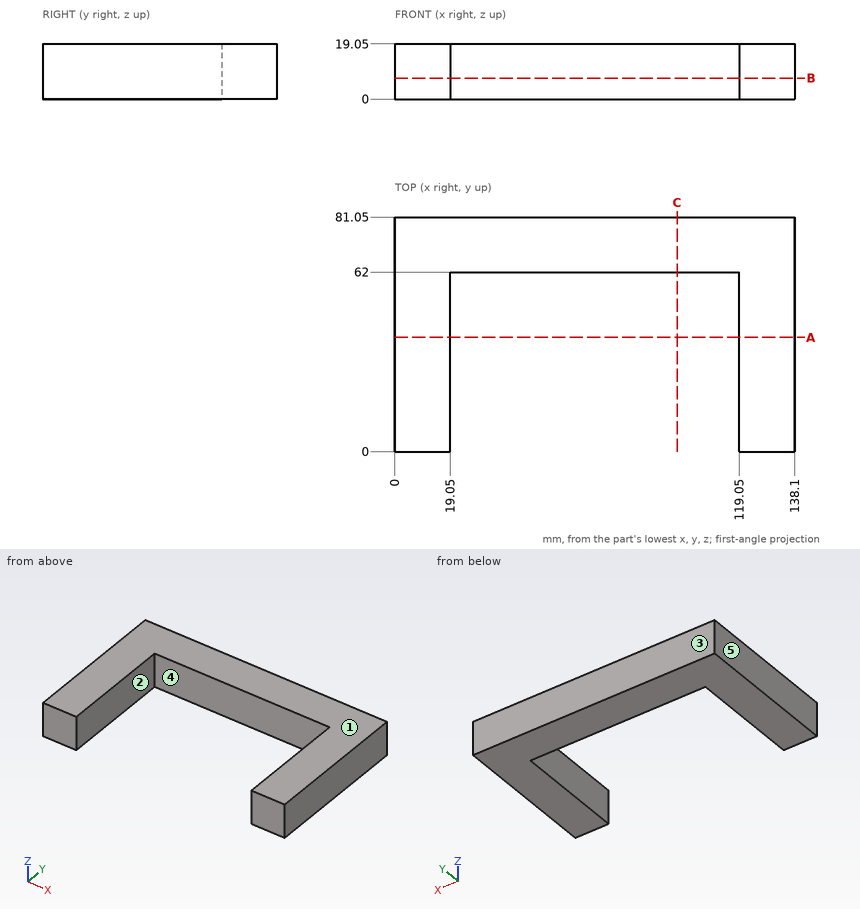
Input: dimensioned drawing with shaded views. Units: mm. Origin: part minimum x, y, z. A direction names the side the tool comes from. Give positions to 0.01 mm unless a question says otherwise; leave off trailing zeros. Order: outer loops, then holes, each group sorted by start corner. A loop starts at its lowest first (then second) coordinate and runs counter-clockwise, first axis right, second up. Notation, with made-up numbers: (4, -6.5) -> (44, -6.5) arc R6 ccw to (44, -2.5) -> close; hole circle Ø1 at (-2.5, 43.5). An arc over 180 degrees is marked (long way). Write item = value, one per line.
Item 1: Section query A-A (y = 39.5). Output: boundary loops of the cut face in (x, z).
Check result:
outline = (0, 0) -> (19.05, 0) -> (19.05, 19.05) -> (0, 19.05) -> close; (119.05, 0) -> (138.1, 0) -> (138.1, 19.05) -> (119.05, 19.05) -> close
Item 2: Section query B-B (z = 7.25). Output: boundary loops of the cut face in (x, y).
Check result:
outline = (0, 0) -> (19.05, 0) -> (19.05, 62) -> (119.05, 62) -> (119.05, 0) -> (138.1, 0) -> (138.1, 81.05) -> (0, 81.05) -> close
Item 3: Contact query for a flat-ended pin moving along its axis: pin 1 (6 mm diameter, centred on x = 51, z = 6, fed in from -Y). Output: stop coordinate, or through.
Check result:
pin_1 = 62
Item 4: Section query C-C (x = 97.5). Output: boundary loops of the cut face in (y, z).
Check result:
outline = (62, 0) -> (81.05, 0) -> (81.05, 19.05) -> (62, 19.05) -> close
Item 5: Set-up query: the marked faces 1 and 2. Return all of +Z, -Z, +X, -X, +Y, -Y with unobstructed straight access to the full face (end or side cutting, diameter ignored); none if empty.
Check result:
face_1 = +Z, +X, -X, +Y, -Y
face_2 = +Z, -Z, -Y
Item 6: Mould query, pull axis X, two halves, no side actions, for the marked faces 3, 4 and 5. Classes: +X half, -X half, draft (parallel to the pull), parting line (faces both ways), or undercut.
Check result:
face_3 = draft
face_4 = undercut
face_5 = -X half
Item 7: Ray query, probe 1 along X at (y, z) = (35, 1.25); probe 2 along Y at (x, z) = (51, 12.75). Return the intervals inside material, ascending.
Check result:
probe_1 = 0 to 19.05, 119.05 to 138.1
probe_2 = 62 to 81.05
